Can you work these out from the model? Positions are in its coordinate system, mm. A direction names the side the tool comes from. Coordinates: 2 decimals unless noted, no trailing zeros. Loops run counter-clockwise (first coordinate to the right, second up) from the corner with the lowest first, then second, coordinate; pieces in that order, holes last. Notation, with made-up numbers: M 8,-29.75 L 19,-29.75 A22 ccw 19,4.25 Z; hole C 9.25,39.5 d10. An arc over 180 degrees is marked long. Answer as a JSON object with one key per item and string values. Group by question number.
Item 1: Suppose I cut it at C-C (y = 27.5). Write out the boundary of the cut face in (x, z).
Item 2: We'd pull the mould along X, two halves only. Please class faces 1 (the flat face through (-15, 11, 3.8)), 2 (the flat face through (15, 11, 3.8)), 3 (the cylindrical face through (1.13, 2.03, 20.23)), 4 (the cylindrical face through (-0.53, 19.62, 2.03)): +X half, -X half, draft (parallel to the pull), parting line (faces both ways), or undercut.
Item 3: Which directions (+Z, -Z, +X, -X, +Y, -Y) give clear straight access to the entire face, cutting with the end or side of a thin tool? Please do faces 5 (the flat face through (-4, 4, 22)), 6 (the flat face through (-0.2, 0, 19.7)).
Item 4: I'm going to push flat-ended pins straight in: pin 1 Ø3 at (x, z) = (11, 33.5) entering from +Y; pin 2 Ø3.5 at (x, z) = (0, 22) entering from +Y. Where does each tip first touch, or does it pass through?
Item 5: Suppose I cut it at D-D (x = -9.5). Write out the boundary of the cut face in (y, z), then the cut area to 3 significant figures.
Item 6: Suppose I cut it at B-B (x = 0). Write out the boundary of the cut face in (y, z).
Item 7: If I drill on line 1 (X direction, y = 1.85, z = 22); line 2 (Y direction, x = 0, z = 1.8); line 3 (Z direction, x = 0, y = 1.05), over which ranges is the centre line in solid material (lowest first)?
Item 8: Suppose I cut it at A-A (z = 22). Write out the boundary of the cut face in (x, y), then the cut area to 3 significant figures.
Autodesk Inventor part; units mm, degrees
ref_plane "YZ Plane" through (0, 0, 0) normal (1, 0, 0) x (0, 1, 0)
ref_plane "XZ Plane" through (0, 0, 0) normal (0, 1, 0) x (-1, 0, 0)
ref_plane "XY Plane" through (0, 0, 0) normal (0, 0, 1) x (1, 0, 0)
sketch "Sketch1" plane through (0, 0, 0) normal (1, 0, 0) x (0, 1, 0)
  line L0 (0, 0) -> (0, 40)
  line L1 (0, 40) -> (4, 40)
  line L2 (4, 40) -> (4, 4)
  line L3 (4, 4) -> (40, 4)
  line L4 (40, 4) -> (40, 0)
  line L5 (40, 0) -> (0, 0)
  dimension "d0" = 40
  dimension "d1" = 4
extrude "Extrusion1" add sketch "Sketch1" along normal mid plane 30
sketch "Sketch4" plane through (-15, 4, 4) normal (0, 0, 1) x (1, 0, 0)
  circle A0 centre (15, 18) radius 2.44
  line L0 (30, 36) -> (30, 0)
  line L1 (0, 36) -> (30, 36)
  point P0 (15, -4)
  point P1 (30, 18)
  point P2 (15, 36)
extrude "Extrusion3" cut sketch "Sketch4" against normal blind 10
sketch "Sketch5" plane through (-15, 4, 40) normal (0, 1, 0) x (1, 0, 0)
  line L0 (0, 0) -> (30, 0)
  line L1 (30, 36) -> (30, 0)
  line L2 (0, 36) -> (30, 36)
  line L3 (0, 0) -> (0, 36)
  circle A0 centre (15, 18) radius 2.1
  point P0 (15, 40)
  point P1 (30, 18)
  point P2 (15, 0)
  dimension "d9" = 4.2
extrude "Extrusion4" cut sketch "Sketch5" against normal through all contours A0
properties part number "30x30_angle" material "Stainless Steel"
From the geometry:
{
 "1": {"outline": "M -15,0 L 15,0 L 15,4 L -15,4 Z"},
 "2": {"face 1": "-X half", "face 2": "+X half", "face 3": "undercut", "face 4": "undercut"},
 "3": {"face 5": "+Z, +X, -X, +Y", "face 6": "+Z, -Z, +X, -X, -Y"},
 "4": {"pin 1": "y = 4", "pin 2": "through"},
 "5": {"outline": "M 0,0 L 40,0 L 40,4 L 4,4 L 4,40 L 0,40 Z", "area": "304 mm2"},
 "6": {"outline": "M 0,0 L 19.56,0 L 19.56,4 L 4,4 L 4,19.9 L 0,19.9 Z; M 0,24.1 L 4,24.1 L 4,40 L 0,40 Z; M 24.44,0 L 40,0 L 40,4 L 24.44,4 Z"},
 "7": {"line 1": "-15 to -2.1, 2.1 to 15", "line 2": "0 to 19.56, 24.44 to 40", "line 3": "0 to 19.9, 24.1 to 40"},
 "8": {"outline": "M -15,0 L -2.1,0 L -2.1,4 L -15,4 Z; M 2.1,0 L 15,0 L 15,4 L 2.1,4 Z", "area": "103 mm2"}
}
